Build history of the part. All positions in model axes, mm. Round coordinates to 2 decimals unless told otherwise and drop trailing zeros. Write each loop counter-clockwise with the first axis right and the second up, starting at its lowest first coordinate (ties: lowest second). Pieces come first, ordered by that corner, then holes. Notation, with made-up numbers: (43, -35.75) -> (89, -35.75) arc R5 cw to (89, -27.75) -> close; hole circle Ø8 at (34.5, 18.5). An arc over 180 degrees is marked (long way). Return JSON: item names as keys, results as strings.
from build123d import *

# Parameters (mm, degrees)
F0_W     = 175.293922
F0_H     = 40.514219
F0_R     = 1.5
F0_R_2   = 1.8288
F0_R_3   = 5.969
F1_DEPTH = 1.70942
F2_R     = 3.69316


with BuildPart() as f1:
    # F0 (on Top) → F1 (new body)
    with BuildSketch(Plane.XY):
        with Locations((0, -2.09611)):
            Rectangle(F0_W, F0_H)
        with Locations((-7.747, -13.418198)):
            Circle(F0_R, mode=Mode.SUBTRACT)
        with Locations((-82.762541, -9.135059)):
            Circle(F0_R_2, mode=Mode.SUBTRACT)
        with Locations((7.747, -13.418198)):
            Circle(F0_R, mode=Mode.SUBTRACT)
        with Locations((0, -7.366)):
            Circle(F0_R_3, mode=Mode.SUBTRACT)
        with Locations((-15.494, 0)):
            Circle(F0_R, mode=Mode.SUBTRACT)
        with Locations((-82.762541, 14.986)):
            Circle(F0_R_2, mode=Mode.SUBTRACT)
        with Locations((-7.747, 13.418198)):
            Circle(F0_R, mode=Mode.SUBTRACT)
        with Locations((15.494, 0)):
            Circle(F0_R, mode=Mode.SUBTRACT)
        with Locations((7.747, 13.418198)):
            Circle(F0_R, mode=Mode.SUBTRACT)
    extrude(amount=F1_DEPTH)

    # F2
    f2_edges = [f1.edges().sort_by_distance(p)[0] for p in [
        (-87.646961, -22.353219, 0.85471),
        (87.646961, -22.353219, 0.85471),
    ]]
    fillet(f2_edges, radius=F2_R)


solid = f1.part
Q1. Saw through at C-C on z = 0.6. Count the separate pieces of the cut face and the enclosed holes in it, then the cut area to 3 significant figures.
Verdict:
{"separate pieces": "1", "enclosed holes": "9", "area": "6,920 mm²"}
Q2. Two-plate mould, pull along X, no slides. Class faces 1 (the cylindrical face through (-1.294, -13.193, 0.843)), 2 (the cylindrical face through (7.55, -11.93, 0.84)), 3 (the cylindrical face through (86.536, -21.3, 0.867)), 4 (the flat face through (-1, 3, 1.709)): +X half, -X half, draft (parallel to the pull), parting line (faces both ways), or undercut.
Verdict:
{"face 1": "undercut", "face 2": "undercut", "face 3": "+X half", "face 4": "draft"}
Q3. Saw through at B-B on y = -4. List the corners of the cut face in (x, z).
Verdict:
{"outline": "(-87.65, 0) -> (-4.93, 0) -> (-4.93, 1.71) -> (-87.65, 1.71) -> close; (4.93, 0) -> (87.65, 0) -> (87.65, 1.71) -> (4.93, 1.71) -> close"}
Q4. Wall check: L1, parallel to X at y = 14, z = 1.55; L2, parallel to Y at x = 0, z = 0.8 (3 decimals); L3, parallel to Y at x = 8.5, z = 1.05. Give the ranges that are in metal, low to high.
Verdict:
{"L1": "x = -87.65 to -84.3, -81.22 to -9.13, -6.36 to 6.36, 9.13 to 87.65", "L2": "y = -22.353 to -13.335, -1.397 to 18.161", "L3": "y = -22.35 to -14.72, -12.12 to 12.12, 14.72 to 18.16"}
Q5. Saw through at A-A on x = 0. List the corners of the cut face in (y, z) (3 decimals).
Verdict:
{"outline": "(-22.353, 0) -> (-13.335, 0) -> (-13.335, 1.709) -> (-22.353, 1.709) -> close; (-1.397, 0) -> (18.161, 0) -> (18.161, 1.709) -> (-1.397, 1.709) -> close"}
